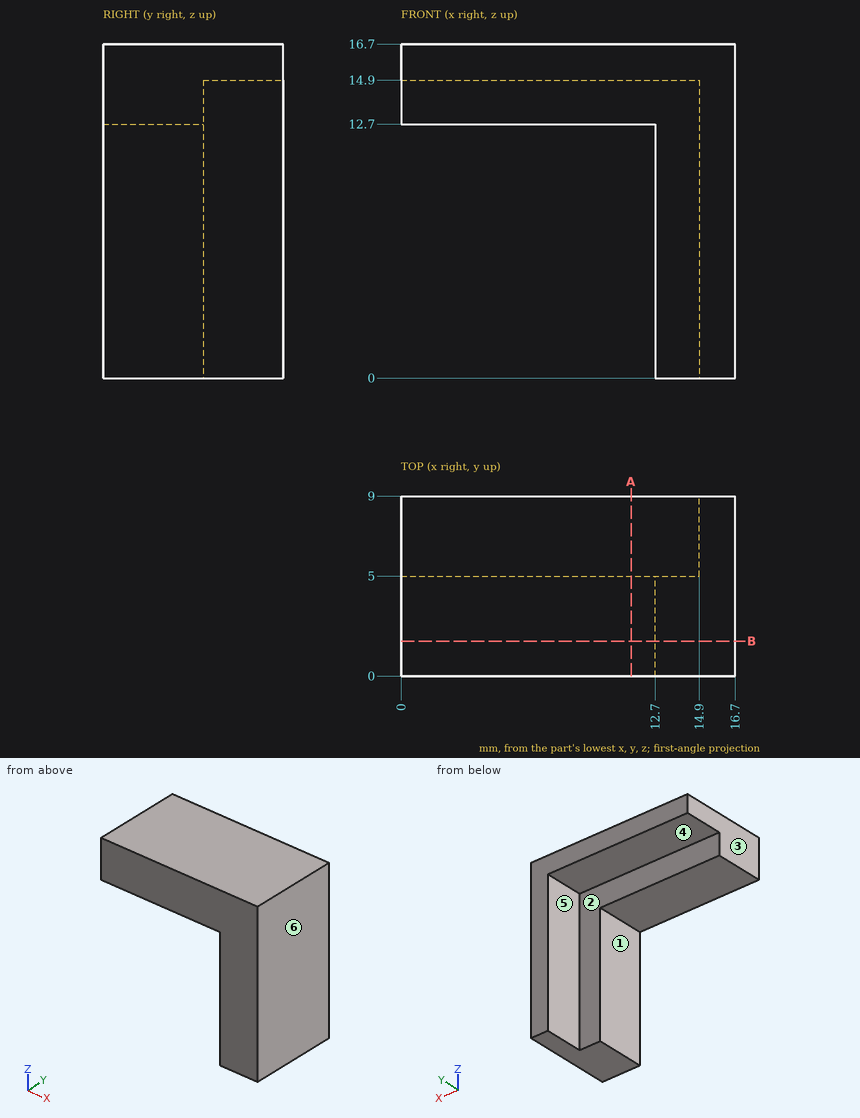
Geometry: see drawing. Coordinates: mm, zero at the bounding-box minimum. A direction names the side the tool comes from. Coordinates: 2 decimals unless noted, no trailing zeros. Loops run counter-clockwise (first coordinate to the right, second up) from the corner with the lowest first, then second, coordinate; pieces in that order, holes last.
Q1. Set-up query: the marked faces 1, 2 and 3. Return all of +Z, -Z, +X, -X, +Y, -Y with unobstructed straight access to the full face (end or side cutting, diameter ignored); none if empty.
Q2. Draft query along X for the marked faces 4, 5 and 6. Return one class per face: +X half, -X half, draft (parallel to the pull), parting line (faces both ways), or undercut.
Q3. Contact query for flat-ended pins moving along their axis: pin 1 (4 mm diameter, centred on y = 3.5, z = 7.5, fed in from -X); pin 2 (1.2 mm diameter, centred on x = 9.5, y = 7.5, fed in from -Z); pin 3 (2.5 mm diameter, centred on x = 8, y = 1.5, fed in from -Z). Output: stop coordinate, or through.
Q4. Cut plane B-B (y = 1.75). Output: boundary loops of the cut face in (x, z), then the cut area to 3 significant figures.
Q5. Material intervals for line 1 (Z direction, x = 3.5, y = 6); line 2 (Z direction, x = 8.25, y = 4), sorted ascending.
Q6. Cut plane A-A (x = 11.5). Output: boundary loops of the cut face in (y, z).
Working result:
1. face 1: -Z, -X, +Y, -Y
1. face 2: -Z, -X, +Y
1. face 3: +Z, -Z, -X, +Y, -Y
2. face 4: draft
2. face 5: -X half
2. face 6: +X half
3. pin 1: stops at x = 12.7
3. pin 2: stops at z = 14.9
3. pin 3: stops at z = 12.7
4. outline: (0, 12.7) - (12.7, 12.7) - (12.7, 0) - (16.7, 0) - (16.7, 16.7) - (0, 16.7) - close
4. area: 118 mm2
5. line 1: z = 14.9 to 16.7
5. line 2: z = 12.7 to 16.7
6. outline: (0, 12.7) - (5, 12.7) - (5, 14.9) - (9, 14.9) - (9, 16.7) - (0, 16.7) - close
